Autodesk Inventor part; units mm, degrees
ref_plane "Work Plane1" through (-47.8335, 6.35, 4.8681) normal (-0.7071, -0.7071, 0) x (0, 0, 1)
ref_plane "Work Plane3" through (-7.1935, 6.35, -35.7719) normal (0.7071, -0.7071, 0) x (0, 0, -1)
ref_plane "YZ Plane" through (0, 0, 0) normal (1, 0, 0) x (0, 1, 0)
sketch "Sketch1" plane through (0, 0, 0) normal (0, 1, 0) x (-1, 0, 0)
  line L0 (7.1935, 4.8681) -> (47.8335, 4.8681)
  line L1 (47.8335, 4.8681) -> (47.8335, -35.7719)
  line L2 (47.8335, -35.7719) -> (7.1935, -35.7719)
  line L3 (7.1935, -35.7719) -> (7.1935, 4.8681)
  point P0 (0, 0)
  point P1 (47.8335, -15.4519)
  dimension "d0" = 40.64
  dimension "d1" = 40.64
extrude "Extrusion1" add sketch "Sketch1" along normal blind 6.35
ref_plane "Work Plane1" through (-47.8335, 6.35, 4.8681) normal (-0.7071, -0.7071, 0) x (0, 0, 1)
sketch "Sketch4" plane through (0, 6.35, 0) normal (0, 1, 0) x (1, 0, 0)
  line L0 (-47.8335, -4.8681) -> (-13.5468, -4.8681)
  line L1 (-47.8335, 35.7719) -> (-7.1935, 35.7719)
  line L2 (-47.8335, -4.8681) -> (-41.4835, -4.8681)
  line L3 (-41.4835, -4.8681) -> (-41.4835, 35.7719)
  line L4 (-41.4835, 35.7719) -> (-47.8335, 35.7719)
  line L5 (-47.8335, 35.7719) -> (-47.8335, -4.8681)
  point P0 (0, 0)
  point P1 (-29.7585, -4.8681)
  dimension "d15" = 6.35
extrude "Extrusion4" add sketch "Sketch4" along normal blind 34.29
sketch "Sketch5" plane through (0, 6.35, 0) normal (0, 1, 0) x (1, 0, 0)
  line L0 (-7.1935, 35.7719) -> (-13.5435, 35.7719)
  line L1 (-13.5435, 35.7719) -> (-13.5435, -4.8681)
  line L2 (-13.5435, -4.8681) -> (-7.1935, -4.8681)
  line L3 (-7.1935, -4.8681) -> (-7.1935, 35.7719)
  line L4 (-7.1935, -4.8681) -> (-7.1935, 35.7719)
  point P0 (0, 0)
  point P1 (-11.6836, 35.7719)
  dimension "d18" = 6.35
  dimension "d19" = 40.64
extrude "Extrusion5" add sketch "Sketch5" along normal blind 34.29
sketch "Sketch6" plane through (-47.8335, 0, 4.8681) normal (0, 0, 1) x (1, 0, 0)
  line L0 (0, 40.64) -> (6.35, 40.64)
  line L1 (0, 40.64) -> (40.64, 40.64)
  line L2 (40.64, 40.64) -> (40.64, 34.29)
  line L3 (40.64, 34.29) -> (0, 34.29)
  line L4 (0, 34.29) -> (0, 40.64)
  point P0 (47.8335, 0)
  dimension "d22" = 40.64
  dimension "d23" = 6.35
extrude "Extrusion6" add sketch "Sketch6" against normal blind 40.64
ref_plane "Work Plane3" through (-7.1935, 6.35, -35.7719) normal (0.7071, -0.7071, 0) x (0, 0, -1)
sketch "Sketch8" plane through (-7.1935, 6.35, -35.7719) normal (0.7071, -0.7071, 0) x (0, 0, -1)
  line L0 (-40.64, -1.3151) -> (-40.64, -7.6651)
  line L1 (-40.64, -4.4901) -> (-40.64, 24.2467)
  line L2 (-40.64, -7.6651) -> (0, -7.6651)
  line L3 (0, -33.2269) -> (0, -4.4901)
  line L4 (0, -7.6651) -> (0, -1.3151)
  line L5 (0, -1.3151) -> (-40.64, -1.3151)
  dimension "d35" = 6.35
extrude "Extrusion7" add sketch "Sketch8" against normal blind 48.4886
sketch "Sketch9" plane through (-47.8335, 6.35, 4.8681) normal (-0.7071, -0.7071, 0) x (0, 0, 1)
  line L0 (0, -4.4901) -> (-40.64, -4.4901)
  line L1 (0, -4.4901) -> (0, -7.6651)
  line L2 (0, -7.6651) -> (-40.64, -7.6651)
  line L3 (-40.64, -7.6651) -> (-40.64, -1.3151)
  line L4 (-40.64, -1.3151) -> (0, -1.3151)
  line L5 (0, -1.3151) -> (0, -4.4901)
  point P0 (-4.8681, -38.3135)
  dimension "d36" = 3.175
  dimension "d37" = 40.64
  dimension "d38" = 90
  dimension "d39" = 6.35
  dimension "d40" = 90
  dimension "d41" = 40.64
  dimension "d42" = 90
extrude "Extrusion8" add sketch "Sketch9" against normal blind 48.4886
sketch "Sketch10" plane through (-7.1935, 0, 4.8681) normal (1, 0, 0) x (0, 0, -1)
  line L0 (0, 0) -> (0, 40.64)
  line L1 (0, 40.64) -> (40.64, 40.64)
  line L2 (40.64, 40.64) -> (40.64, 0)
  line L3 (40.64, 0) -> (0, 0)
  line L4 (0, 0) -> (0, 40.64)
  point P0 (4.8681, 0)
extrude "Extrusion9" cut sketch "Sketch10" against normal blind 3.175
mirror "Mirror1" about plane through (-10.3685, 20.32, -15.4519) normal (1, 0, 0)
sketch "Sketch11" plane through (27.0965, 0, 4.8681) normal (1, 0, 0) x (0, 0, -1)
  line L0 (0, 40.64) -> (40.64, 40.64)
  line L1 (40.64, 40.64) -> (40.64, 0)
  line L2 (40.64, 0) -> (0, 0)
  line L3 (0, 0) -> (0, 40.64)
  point P0 (4.8681, 0)
  dimension "d47" = 40.64
  dimension "d48" = 40.64
extrude "Extrusion10" cut sketch "Sketch11" against normal blind 3.175
mirror "Mirror2" about plane through (23.9215, 20.32, -15.4519) normal (1, 0, 0)
sketch "Sketch12" plane through (-47.8335, 0, 4.8681) normal (0, 0, 1) x (1, 0, 0)
  circle A0 centre (-25.4, 20.32) radius 6.35
  line L0 (143.51, 40.64) -> (0, 40.64)
  line L1 (0, 0) -> (0, 40.64)
  line L2 (-19.3329, 30.0069) -> (0, 40.64)
  line L3 (-19.3329, 10.6331) -> (0, 0)
  arc A1 (-19.3329, 30.0069) -> (-19.3329, 10.6331) centre (-25.4, 20.32) ccw
  point P0 (47.8335, 0)
  dimension "d51" = 12.7
  dimension "d52" = 20.32
  dimension "d53" = 25.4
  dimension "d54" = 22.86
extrude "Extrusion11" add sketch "Sketch12" against normal blind 40.64
properties part number "Leg Box"
Geometry: final body of the model. Coordinates: model frame, mm. A direction names the side the tool comes from. Round coordinates to 2 decimals unless told otherwise and drop trailing zeros. Order: outer loops, then holes, each group sorted by start corner. A loop starts at its lowest first (then second) coordinate and runs counter-clockwise, first axis right, second up. Notation, with made-up numbers: (84, 55.25) -> (112, 55.25) arc R9 ccw to (112, 67.25) -> close; hole circle Ø2 at (-4.75, 79.25). An arc over 180 degrees is marked (long way). Put each result on its own line as item: value. Start each with the question number.
Q1. Reachability of faces 1 (the flat face through (70.55, 11.024, -15.736)), 2 (the flat face through (4, 21, 4.868)) from +Z, -Z, +X, -X, +Y, -Y: full face, straight path, thin tool, end or side. Return the list, or none.
Q2. Line query: probe 1 along Y at (x, z) = (83.5, -29); probe 2 along Y at (x, z) = (0, -30.5); probe 3 along Y at (x, z) = (-24, -27). Output: solid intervals per line, ascending.
Q3. Section B-B on z = -3. Give the number of separate pieces and of enclosed holes in the cut face, and give its area (3 significant figures).
Q4. Section A-A on x = 29. Return the cut outline in (y, z), and give its area (3 significant figures).
Q5. First-contact query: pin 1 (5 mm diameter, centred on y = 13.5, z = -3, fed in from -X); pin 2 (5.5 mm diameter, centred on y = 17, z = -8.5, fed in from -X); pin 3 (8 mm diameter, centred on y = 6, z = -30.5, fed in from -X). Flat tips, straight axial feed; report the tip coordinate or a pass-through.
Q6. Pull-direction query (Y, two-part tool) for faces 3 (the flat face through (45.74, 29.484, -15.736)), 4 (the flat face through (-41.484, 20, -15)), 5 (the flat face through (4, 21, -35.772)), 6 (the flat face through (23, 40.64, -16)); classes: +Y half, -Y half, draft (parallel to the pull), parting line (faces both ways), or undercut.
Ans:
1. face 1: +Z, -Z
1. face 2: +Z, +X, -X, +Y, -Y
2. probe 1: y = 0 to 6.35, 7.69 to 16.67, 23.97 to 32.95, 34.29 to 40.64
2. probe 2: y = 0 to 6.35, 9.05 to 18.03, 22.61 to 31.59, 34.29 to 40.64
2. probe 3: y = 0 to 6.35, 12.32 to 28.32, 34.29 to 40.64
3. separate pieces: 1
3. enclosed holes: 17
3. area: 5,180 mm2
4. outline: (0, -35.77) -> (12.74, -35.77) -> (12.74, 4.87) -> (0, 4.87) -> close; (27.9, -35.77) -> (40.64, -35.77) -> (40.64, 4.87) -> (27.9, 4.87) -> close
4. area: 1,040 mm2
5. pin 1: stops at x = -83.82
5. pin 2: stops at x = -84.65
5. pin 3: stops at x = -78.15
6. face 3: undercut
6. face 4: undercut
6. face 5: draft
6. face 6: +Y half
